Can you work these out from the model? Positions are in its coordinate system, mm. Coordinates: 2 decimals unless noted, no trailing zeros. Write each loop counter-clockwise with the first axis right and the second up, starting at its lowest first coordinate (ties: lowest second). Pieces come first, ordered by that corner, then holes.
```python
from build123d import *

# Parameters (mm, degrees)
SKETCH1_W           = 1120
SKETCH1_H           = 180
SKETCH1_W_2         = 1100
SKETCH1_H_2         = 170
BOSS_EXTRUDE1_DEPTH = 1
SKETCH2_R           = 1
BOSS_EXTRUDE2_DEPTH = 2


with BuildPart() as part:
    # Sketch1 → Boss-Extrude1 (new body)
    with BuildSketch(Plane.XY):
        Rectangle(SKETCH1_W, SKETCH1_H)
        Rectangle(SKETCH1_W_2, SKETCH1_H_2, mode=Mode.SUBTRACT)
    extrude(amount=BOSS_EXTRUDE1_DEPTH)

    # Sketch2 → Boss-Extrude2 (add)
    with BuildSketch(Plane.XY.offset(1)):
        with Locations((-555, 0)):
            Circle(SKETCH2_R)
    boss_extrude2 = extrude(amount=BOSS_EXTRUDE2_DEPTH)

    # Mirror1: Boss-Extrude2 across plane
    add(boss_extrude2.mirror(Plane(origin=(0, 0, 0), x_dir=(0, 0, 1), z_dir=(1, 0, 0))))


solid = part.part
```
1. If we section it at B-B, the plane x = 475: List the corners of the cut face in (y, z) for me.
2. If I drill on L1, parallel to Y at x = -330.5, z = 0.3; L2, parallel to X at y = 47.5, z = 0.25, over which ranges is the centre line in solid material (lowest first)?
3. If we section it at A-A, the plane y = 14.5: List the corners of the cut face in (x, z) for me, plus the area to 3 significant figures.
Answers:
1. outline: (-90, 0) - (-85, 0) - (-85, 1) - (-90, 1) - close; (85, 0) - (90, 0) - (90, 1) - (85, 1) - close
2. L1: y = -90 to -85, 85 to 90
2. L2: x = -560 to -550, 550 to 560
3. outline: (-560, 0) - (-550, 0) - (-550, 1) - (-560, 1) - close; (550, 0) - (560, 0) - (560, 1) - (550, 1) - close
3. area: 20.0 mm2
